from build123d import *

# Parameters (mm, degrees)
Y_KSEKLIK_EKSTR_ZYON1_DEPTH = 50
IZIM2_R                     = 1.6
KES_EKSTR_ZYON1_DEPTH       = 57.391488719


with BuildPart() as part:
    # Çizim1 → Yükseklik-Ekstrüzyon1 (new body)
    with BuildSketch(Plane.XY):
        with BuildLine():
            Line((-8, 0), (-22, 0))
            Line((-22, 0), (-22, 14))
            Line((-22, 14), (22, 14))
            Line((22, 14), (22, 0))
            Line((22, 0), (8, 0))
            ThreePointArc((8, 0), (0, 8), (-8, 0))
        make_face()
    extrude(amount=-Y_KSEKLIK_EKSTR_ZYON1_DEPTH)

    # Çizim2 → Kes-Ekstrüzyon1 (cut, through all)
    with BuildSketch(Plane(origin=(0, 14, 0), x_dir=(1, 0, 0), z_dir=(0, 1, 0))):
        with Locations(Location((-15, 25, 0), (0, 0, 180))):
            Circle(IZIM2_R)
        with Locations(Location((-15, 37.5, 0), (0, 0, 180))):
            Circle(IZIM2_R)
        with Locations(Location((-15, 12.5, 0), (0, 0, 180))):
            Circle(IZIM2_R)
        with Locations((15, 12.5)):
            Circle(IZIM2_R)
        with Locations((15, 37.5)):
            Circle(IZIM2_R)
        with Locations((15, 25)):
            Circle(IZIM2_R)
    extrude(amount=-KES_EKSTR_ZYON1_DEPTH, mode=Mode.SUBTRACT)


solid = part.part
For this review, take the finished solid that the model builds, in its own axes (mm). Coordinates: 2 decimals unless noted, no trailing zeros. Loops run counter-clockwise (first coordinate to the right, second up) from the corner with the lowest first, then second, coordinate; pieces in that order, holes last. Notation, with made-up numbers: (-40, 13) - (9, 13) arc R22 cw to (9, 48) - close; hole circle Ø3 at (33, -0.5). An arc over 180 degrees is marked (long way). Use a Markdown table: item, result. Add a question column.
Item 1: We need section B-B (x = -15). Give the boundary of the cut face in (y, z).
Item 2: We need section A-A (z = -12.5). Give the boundary of the cut face in (x, y), and give its area (3 significant figures).
Item 3: Mouldability with a two-part tool opening along Z and no side actions: class faces 1 (the face through (0, 9, 0)), 2 (the face through (-22, 7, -25)), 3 (the face through (13.73, 7.1, -36.53)) as pulls with the +Z half, pulls with the -Z half, needs draft (parallel to the pull), parting line crosses it, or undercut.
Item 4: We need section D-D (z = -46). Give the boundary of the cut face in (x, y).
Item 5: We need section C-C (y = 10.5). Give the boundary of the cut face in (x, z).
Item 6: For line 1 (Z direction, x = 15, y = 9.25); line 2 (X direction, y = 4.75, z = -26); line 3 (X direction, y = 4.75, z = -17), list the stretches that pass through material, from the lowest coordinate up.
Results list:
| question | item | result |
|---|---|---|
| 1 | outline | (0, -50) - (14, -50) - (14, -39.1) - (0, -39.1) - close; (0, -35.9) - (14, -35.9) - (14, -26.6) - (0, -26.6) - close; (0, -23.4) - (14, -23.4) - (14, -14.1) - (0, -14.1) - close; (0, -10.9) - (14, -10.9) - (14, 0) - (0, 0) - close |
| 2 | outline | (-22, 0) - (-16.6, 0) - (-16.6, 14) - (-22, 14) - close; (-13.4, 0) - (-8, 0) arc R8 cw to (8, 0) - (13.4, 0) - (13.4, 14) - (-13.4, 14) - close; (16.6, 0) - (22, 0) - (22, 14) - (16.6, 14) - close |
| 2 | area | 426 mm^2 |
| 3 | face 1 | pulls with the +Z half |
| 3 | face 2 | needs draft |
| 3 | face 3 | undercut |
| 4 | outline | (-22, 0) - (-8, 0) arc R8 cw to (8, 0) - (22, 0) - (22, 14) - (-22, 14) - close |
| 5 | outline | (-22, -50) - (22, -50) - (22, 0) - (-22, 0) - close; hole circle Ø3.2 at (-15, -37.5); hole circle Ø3.2 at (-15, -25); hole circle Ø3.2 at (-15, -12.5); hole circle Ø3.2 at (15, -37.5); hole circle Ø3.2 at (15, -25); hole circle Ø3.2 at (15, -12.5) |
| 6 | line 1 | z = -50 to -39.1, -35.9 to -26.6, -23.4 to -14.1, -10.9 to 0 |
| 6 | line 2 | x = -22 to -16.25, -13.75 to -6.44, 6.44 to 13.75, 16.25 to 22 |
| 6 | line 3 | x = -22 to -6.44, 6.44 to 22 |
